Part print with two shaded views. Sizes in mm from the minimum x, y, z corner. A direction names the side the tool comes from. Round coordinates to 2 decimals unless told otherwise and drop trailing zeros. Order: outer loops, then holes, each group sorted by start corner. A loop starts at its lowest first (then second) coordinate and runs counter-clockwise, first axis right, second up. Notation, with made-up numbers: (43, 6) -> (70, 6) arc R21 cw to (70, 13) -> close; hole circle Ø9 at (87, -13). An arc over 180 degrees is marked (long way). Use a Markdown table: item, result. Add a question column.
Item 1: Slice it at A-A, the plane y = 2.75. Give the cut face in (x, z), plus the area to 3 significant figures.
Item 2: Slice it at B-B, the plane z = 6. Give the cut face in (x, y).
Item 3: 3-axis set-ups, long thin cutter, end or side, ignore diameter. For the marked faces 1, 2 and 3: which of +Z, -Z, +X, -X, +Y, -Y reach the whole face in a straight line?
Item 4: Pin check, flat tips, straight feed: pin 1 (2 mm diameter, centred on x = 7.5, y = 0.5, fed in from -Z); pin 2 (1 mm diameter, centred on x = 7, z = 2, fed in from +Y); pin 3 (4 mm diameter, centred on x = 4.5, z = 5, fed in from +Y). Stop position of each tip, or through.
Item 5: Probe L1, parallel to Z at x = 1.75, y = 5.25; L2, parallel to X at y = 5, z = 4.75; L3, parallel to Y at x = 3.5, z = 4. List the from-to ranges inside material, lowest first.
Item 6: Slice it at D-D, the plane z = 3.5. Give the cut face in (x, y), plus the area to 3 significant figures.
Item 7: Slice it at C-C, the plane x = 1.5. Give the cut face in (y, z), plus the area to 3 significant figures.
Item 8: Two-plate mould, pull along X, no slides. Class the marked faces 4, 5, 6 and 7: released by +X, released by -X, zero draft, split by the parting line, or undercut.
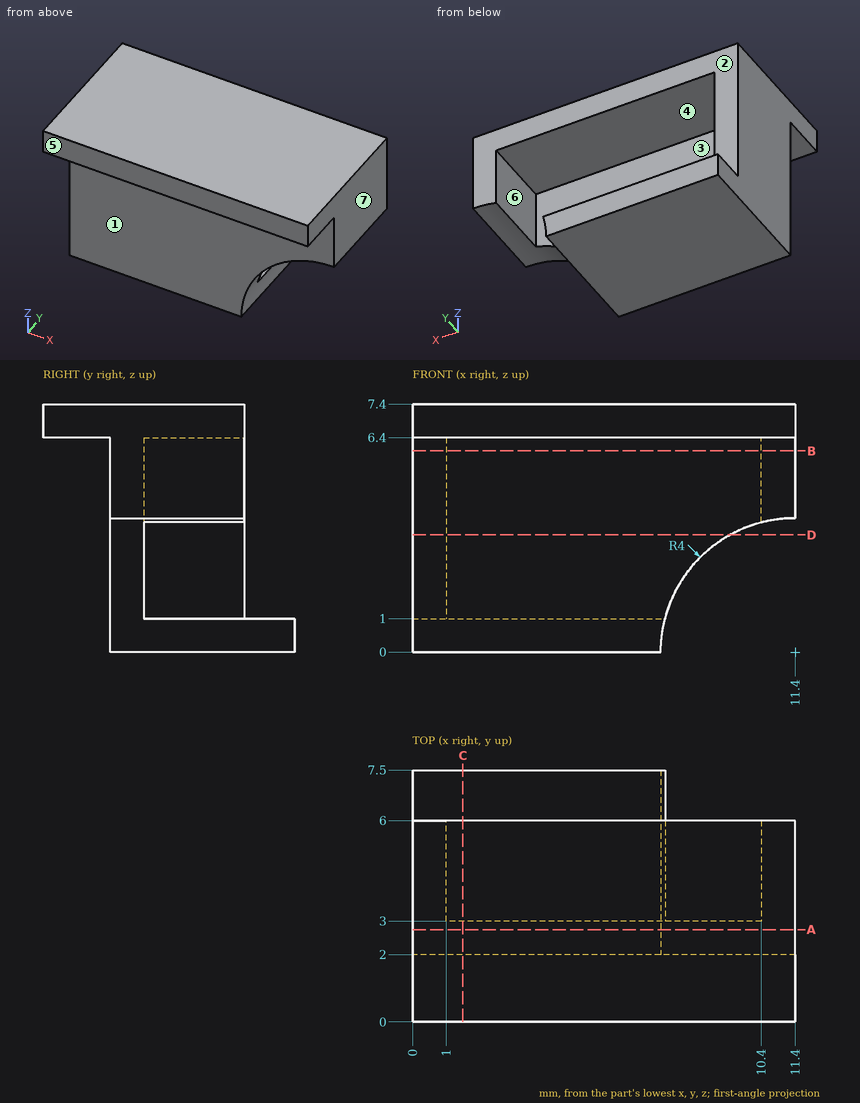
Check sheet entries:
| question | item | result |
|---|---|---|
| 1 | outline | (0, 0) -> (7.4, 0) arc R4 cw to (11.4, 4) -> (11.4, 7.4) -> (0, 7.4) -> close |
| 1 | area | 71.8 mm2 |
| 2 | outline | (0, 2) -> (11.4, 2) -> (11.4, 6) -> (10.4, 6) -> (10.4, 3) -> (1, 3) -> (1, 6) -> (0, 6) -> close |
| 3 | face 1 | -Z, +X, -X, -Y |
| 3 | face 2 | +Z, +X, -X, +Y |
| 3 | face 3 | +Y |
| 4 | pin 1 | z = 6.4 |
| 4 | pin 2 | y = 3 |
| 4 | pin 3 | y = 6 |
| 5 | L1 | 0 to 1, 6.4 to 7.4 |
| 5 | L2 | 0 to 1, 10.4 to 11.4 |
| 5 | L3 | 2 to 3 |
| 6 | outline | (0, 2) -> (9.46, 2) -> (9.46, 3) -> (1, 3) -> (1, 6) -> (0, 6) -> close |
| 6 | area | 12.5 mm2 |
| 7 | outline | (0, 6.4) -> (2, 6.4) -> (2, 0) -> (7.5, 0) -> (7.5, 1) -> (3, 1) -> (3, 6.4) -> (6, 6.4) -> (6, 7.4) -> (0, 7.4) -> close |
| 7 | area | 16.9 mm2 |
| 8 | face 4 | undercut |
| 8 | face 5 | zero draft |
| 8 | face 6 | undercut |
| 8 | face 7 | released by +X |
